```python
from build123d import *

# Parameters (mm, degrees)
SKETCH1_W            = 53
SKETCH1_H            = 50
BOSS_EXTRUDE1_DEPTH  = 3
CUT_EXTRUDE1_DEPTH   = 73.924618614
SKETCH3_W            = 3
SKETCH3_H            = 50
BOSS_EXTRUDE2_DEPTH  = 48
SKETCH4_R            = 11.05
CUT_EXTRUDE2_DEPTH   = 89.938180777
M3_CLEARANCE_HOLE1_D = 3.4
M3_CLEARANCE_HOLE2_D = 3.4
CHAMFER1_SIZE        = 5.08


with BuildPart() as part:
    # Sketch1 → Boss-Extrude1 (new body)
    with BuildSketch(Plane.XY):
        with Locations((26.5, 25)):
            Rectangle(SKETCH1_W, SKETCH1_H)
    extrude(amount=BOSS_EXTRUDE1_DEPTH)

    # Sketch2 → Cut-Extrude1 (cut, through all)
    with BuildSketch(Plane.XY.offset(3)):
        with BuildLine():
            Line((42, 37.9), (12, 37.9))
            ThreePointArc((12, 37.9), (9.9, 40), (12, 42.1))
            Line((12, 42.1), (42, 42.1))
            ThreePointArc((42, 42.1), (44.1, 40), (42, 37.9))
        make_face()
        with BuildLine():
            Line((42, 12.1), (12, 12.1))
            ThreePointArc((12, 12.1), (9.9, 10), (12, 7.9))
            Line((12, 7.9), (42, 7.9))
            ThreePointArc((42, 7.9), (44.1, 10), (42, 12.1))
        make_face()
    extrude(amount=-CUT_EXTRUDE1_DEPTH, mode=Mode.SUBTRACT)

    # Sketch3 → Boss-Extrude2 (add)
    with BuildSketch(Plane.XY.offset(3)):
        with Locations((1.5, 25)):
            Rectangle(SKETCH3_W, SKETCH3_H)
    extrude(amount=BOSS_EXTRUDE2_DEPTH)

    # Sketch4 → Cut-Extrude2 (cut, through all)
    with BuildSketch(Plane.ZY):
        with Locations((30, 25)):
            Circle(SKETCH4_R)
    extrude(amount=-CUT_EXTRUDE2_DEPTH, mode=Mode.SUBTRACT)

    # M3 Clearance Hole1 (through all)
    with Locations(Plane.ZY):
        with Locations((45.5, 9.5), (14.5, 40.5), (14.5, 9.5), (45.5, 40.5)):
            Hole(M3_CLEARANCE_HOLE1_D / 2)

    # M3 Clearance Hole2 (through all)
    with Locations(Plane.ZY):
        with Locations((39.899494937, 34.899494937), (39.899494937, 15.100505063), (20.100505063, 34.899494937), (20.100505063, 15.100505063)):
            Hole(M3_CLEARANCE_HOLE2_D / 2)

    # Chamfer1
    chamfer1_edges = [part.edges().sort_by_distance(p)[0] for p in [
        (1.5, 0, 51),
        (1.5, 50, 51),
        (53, 50, 1.5),
        (53, 0, 1.5),
    ]]
    chamfer(chamfer1_edges, length=CHAMFER1_SIZE)


solid = part.part
```
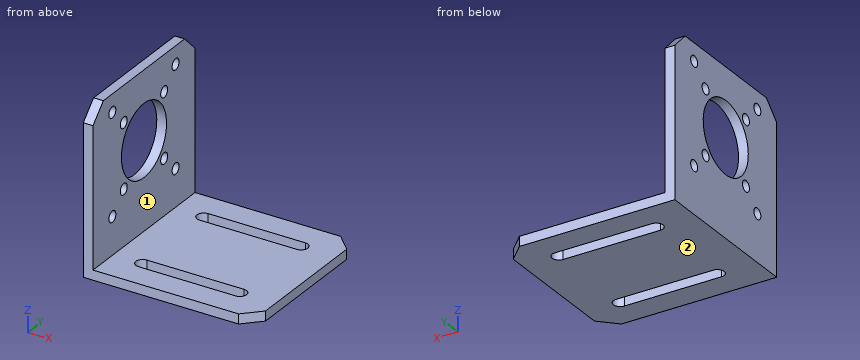
Can you work these out from the model? Positions are in its coordinate system, mm. Face numbers are marked on the shaded views. A direction names the side the tool comes from. Give positions to 0.01 mm unless a question says otherwise; leave off trailing zeros. Loops run counter-clockwise (first coordinate to the right, second up) from the corner with the lowest first, then second, coordinate; pieces in that order, holes last. Notation, with made-up numbers: M 0.5,28.25 L 6.5,28.25 A20 ccw 6.5,41.25 Z; hole C 69,20.5 d1. An arc over 180 degrees is marked long. One line per item, written item: value.
(1) Suppose I cut it at A-A on z = 14.5. List the corners of the cut face in (x, y) for me.
Returned:
outline: M 0,0 L 3,0 L 3,7.8 L 0,7.8 Z; M 0,11.2 L 3,11.2 L 3,38.8 L 0,38.8 Z; M 0,42.2 L 3,42.2 L 3,50 L 0,50 Z
(2) Which directions (+Z, -Z, +X, -X, +Y, -Y) give clear straight access to the entire face, cutting with the end or side of a thin tool? Please do the marked faces 1 and 2.
Returned:
face 1: +Z, +X, +Y, -Y
face 2: -Z, +X, -X, +Y, -Y
(3) Will these pins go through, and if not, where does the flat tip stop? pin 1 (4 mm diameter, centred on y = 15.1, z = 20.1, fed in from -X); pin 2 (2 mm diameter, centred on y = 31.5, z = 21, fed in from +X); pin 3 (4 mm diameter, centred on x = 6, y = 29.5, fed in from +Z).
Returned:
pin 1: x = 0
pin 2: x = 3
pin 3: z = 3
(4) Suppose I cut it at B-B on x = 25.5. List the corners of the cut face in (y, z) for me, plus the area to 3 significant figures.
Returned:
outline: M 0,0 L 7.9,0 L 7.9,3 L 0,3 Z; M 12.1,0 L 37.9,0 L 37.9,3 L 12.1,3 Z; M 42.1,0 L 50,0 L 50,3 L 42.1,3 Z
area: 125 mm^2
(5) I need wall thicknesses on line 1 (Y direction, x = 1.2, z = 14.5); line 2 (X direction, y = 31, z = 13.5). Which ranges of each line are inside material? Lowest first, please.
Returned:
line 1: 0 to 7.8, 11.2 to 38.8, 42.2 to 50
line 2: 0 to 3
(6) Suppose I cut it at D-D on z = 25.5. List the corners of the cut face in (x, y) for me, plus the area to 3 significant figures.
Returned:
outline: M 0,0 L 3,0 L 3,14.91 L 0,14.91 Z; M 0,35.09 L 3,35.09 L 3,50 L 0,50 Z
area: 89.4 mm^2
(7) Suppose I cut it at C-C on y = 40.5. List the corners of the cut face in (x, z) for me, plus the area to 3 significant figures.
Returned:
outline: M 0,0 L 9.96,0 L 9.96,3 L 3,3 L 3,12.8 L 0,12.8 Z; M 0,16.2 L 3,16.2 L 3,43.8 L 0,43.8 Z; M 0,47.2 L 3,47.2 L 3,51 L 0,51 Z; M 44.04,0 L 53,0 L 53,3 L 44.04,3 Z
area: 180 mm^2
